```python
from build123d import *

# Parameters (mm, degrees)
F1_DEPTH = 3
F0_W     = 4.5
F0_H     = 7
F2_DEPTH = 23
F0_W_2   = 25
F0_H_2   = 3
F3_DEPTH = 26
F4_R     = 8.75
F5_DEPTH = 2
F6_R     = 2
F7_W     = 25
F7_H     = 3
F8_DEPTH = 20
F9_R     = 5


with BuildPart() as f1:
    # F0 (on Front) → F1 (new body)
    with BuildSketch(Plane.XZ):
        Polygon((4.5, 7), (4.5, 0), (20.5, 0), (20.5, 7), (25, 7), (25, 22), (0, 22), (0, 7), align=None)
    extrude(amount=F1_DEPTH)

    # F0 (on Front) → F2 (join)
    with BuildSketch(Plane.XZ):
        with Locations((2.25, 3.5)):
            Rectangle(F0_W, F0_H)
        with Locations((22.75, 3.5)):
            Rectangle(F0_W, F0_H)
    extrude(amount=F2_DEPTH)

    # F0 (on Front) → F3 (join)
    with BuildSketch(Plane.XZ):
        with Locations((12.5, 23.5)):
            Rectangle(F0_W_2, F0_H_2)
    extrude(amount=F3_DEPTH)

    # F4 (on face) → F5 (join)
    with BuildSketch(Plane.XY.offset(25)):
        with Locations((12.5, -13)):
            Circle(F4_R)
    extrude(amount=F5_DEPTH)

    # F6
    f6_edges = [f1.edges().sort_by_distance(p)[0] for p in [
        (0, -13, 25),
        (25, -13, 25),
        (0, -11.5, 0),
        (25, -11.5, 0),
    ]]
    fillet(f6_edges, radius=F6_R)

    # F7 (on face) → F8 (join, through all)
    with BuildSketch(Plane.XZ.offset(23)):
        with Locations((12.5, 8.5)):
            Rectangle(F7_W, F7_H)
    extrude(amount=-F8_DEPTH)

    # F9
    f9_edges = [f1.edges().sort_by_distance(p)[0] for p in [
        (12.5, -3, 10),
        (12.5, -3, 22),
    ]]
    fillet(f9_edges, radius=F9_R)


solid = f1.part
```
Geometry check sheet. Reference: the model listing, model coordinates, mm. A direction names the side the tool comes from. Coordinates: 2 decimals unless noted, no trailing zeros. Order: outer loops, then holes, each group sorted by start corner. A loop starts at its lowest first (then second) coordinate and runs counter-clockwise, first axis right, second up. Notation, with made-up numbers: M 77,48 L 109,48 A21 ccw 109,78 Z; hole C 7.5,49.25 d1. An arc over 180 degrees is marked long. One line per question, with ' | ' between items. Start each with the question number.
Item 1: Cross-section at C-C on z = 4.25. Enter the section's corners in (x, y), then the cut area to 3 significant figures.
Item 2: Cross-section at A-A on y = -13. Enter the section's corners in (x, z).
Item 3: Cross-section at D-D on y = -1.75. Enter the section's corners in (x, z), then the cut area to 3 significant figures.
Item 4: Material ranges on L1, parallel to Z at x = 15.75, y = -19.25; L2, parallel to Z at x = 18.5, y = -21.25; L3, parallel to X at y = -14.5, z = 6.5, recorded low to high. Write a range as [from, to].
Item 5: Draft check along X on faces 5 (the flat face through (12, -13, 7)), 6 (the cylindrical face through (24.4, -11.66, 0.57)), 7 (the flat face through (12, -17, 22)). Enter one of: pulls with the +X half, pulls with the -X half, needs draft (parallel to the pull), parting line crosses it, or undercut.
Item 6: Gauge pin test, flat ends, axial feed: pin 1 (3.5 mm diameter, centred on x = 9, z = 2.5, fed in from -Y); pin 2 (2 mm diameter, centred on x = 16, y = -21, fed in from -Z); pin 3 (4 mm diameter, centred on y = -20.5, z = 13, fed in from -X). Record the tip position at first contact, or that the pin passes through.
Item 7: Cross-section at B-B on x = 12.5. Enter the section's corners in (y, z), then the cut area to 3 significant figures.
Item 8: Set-up check for faces 1 (the cylindrical face through (12, -4, 20)), 2 (the flat face through (12, -2, 0)), 3 (the flat face through (12, -4, 25)), 4 (the flat face through (4.5, -13, 3)): record each of +Z, -Z, +X, -X, +Y, -Y from which the full face is reachable in a straight line by a thin tool's end or side.
Findings:
1) outline: M 0,-23 L 4.5,-23 L 4.5,-3 L 20.5,-3 L 20.5,-23 L 25,-23 L 25,0 L 0,0 Z | area: 255 mm²
2) outline: M 0,2 A2 ccw 2,0 L 4.5,0 L 4.5,7 L 20.5,7 L 20.5,0 L 23,0 A2 ccw 25,2 L 25,10 L 0,10 Z; M 0,22 L 25,22 L 25,23 A2 ccw 23,25 L 21.25,25 L 21.25,27 L 3.75,27 L 3.75,25 L 2,25 A2 ccw 0,23 Z
3) outline: M 0,2 A2 ccw 2,0 L 23,0 A2 ccw 25,2 L 25,23 A2 ccw 23,25 L 2,25 A2 ccw 0,23 Z | area: 622 mm²
4) L1: z = [7, 10], [22, 27] | L2: z = [7, 10], [22, 25] | L3: x = [0, 4.5], [20.5, 25]
5) face 5: undercut | face 6: pulls with the +X half | face 7: needs draft
6) pin 1: stops at y = -3 | pin 2: stops at z = 7 | pin 3: passes through
7) outline: M -26,22 L -8,22 A5 cw -3,17 L -3,15 A5 cw -8,10 L -23,10 L -23,7 L -3,7 L -3,0 L 0,0 L 0,25 L -4.25,25 L -4.25,27 L -21.75,27 L -21.75,25 L -26,25 Z | area: 250 mm²
8) face 1: +X, -X, -Y | face 2: -Z, +X, -X, +Y, -Y | face 3: +Z | face 4: -Z, -Y
